Drawing for the job (mm, zero at the part's lowest x, y, z). Give positions to 0.01 mm unless a question says otherwise; leave off trailing zeros. Loops run counter-clockwise (first coordinate to the right, second up) from the corner with the lowest first, then second, coordinate; pieces in that order, holes last. Notation, with made-up numbers: M -8.5,-8 L 41.5,-8 A5 cw 41.5,-4 Z; hole C 85.25,65.25 d3. An arc over 180 degrees is marked long. Use CSV: the item, a comma, the result in double quotes. Start each with the question number.
(1) Wall check: line 1 along X through (y, z) = (28, 3.35) (1 decimal); line 2 along X through (y, z) = (22, 5.75) (1 decimal); line 3 along Y through (x, z) = (28, 4.7). Give the ranges that are in metal, low to high. Write a range as from..to.
(2) Slice it at A-A on z = 2.5. List the corners of the cut face in (x, y) (1 decimal), and give its area (3 significant figures).
(3) Slice it at C-C on x = 27.5. List the corners of the cut face in (y, z).
(4) Slice it at B-B on y = 30. List the corners of the cut face in (x, z), and give its area (3 significant figures).
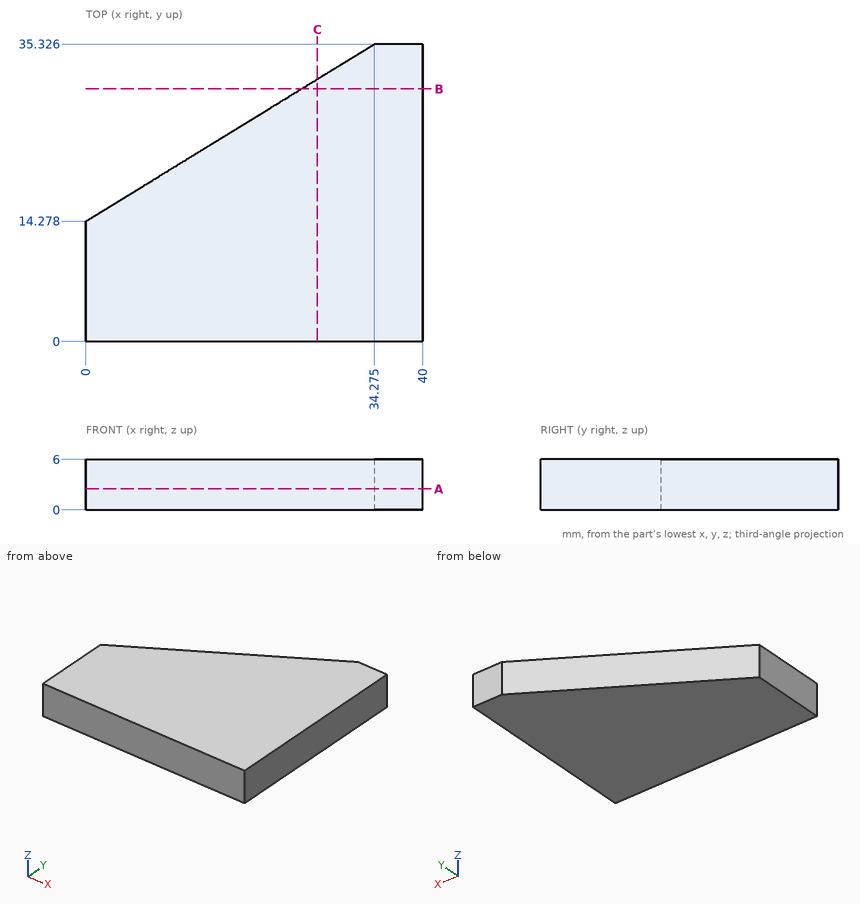
Reply:
1,line 1,"x = 22.3..40"
1,line 2,"x = 12.6..40"
1,line 3,"y = 0..31.47"
2,outline,"M 0,0 L 40,0 L 40,35.3 L 34.3,35.3 L 0,14.3 Z"
2,area,"1,050 mm^2"
3,outline,"M 0,0 L 31.17,0 L 31.17,6 L 0,6 Z"
4,outline,"M 25.6,0 L 40,0 L 40,6 L 25.6,6 Z"
4,area,"86.4 mm^2"
